```python
from build123d import *

# Parameters (mm, degrees)
SKETCH1_R           = 1.5
SKETCH1_R_2         = 53.34
BOSS_EXTRUDE1_DEPTH = 1.5875
CUT_EXTRUDE3_DEPTH  = 140.70900378


with BuildPart() as part:
    # Sketch1 → Boss-Extrude1 (new body)
    with BuildSketch(Plane(origin=(0, 0, 0), x_dir=(1, 0, 0), z_dir=(0, 1, 0))):
        Polygon((0.047005036, -98.782806148), (-98.782806148, -0.047005036), (-0.047005036, 98.782806148), (98.782806148, 0.047005036), align=None)
        with Locations(Location((-61.346730494, 5.55625, 0), (0, 0, 270))):
            Circle(SKETCH1_R, mode=Mode.SUBTRACT)
        with Locations(Location((-61.346730494, -5.55625, 0), (0, 0, 270))):
            Circle(SKETCH1_R, mode=Mode.SUBTRACT)
        with Locations(Location((-5.55625, -61.346730494, 0), (0, 0, 270))):
            Circle(SKETCH1_R, mode=Mode.SUBTRACT)
        with Locations(Location((5.55625, -61.346730494, 0), (0, 0, 270))):
            Circle(SKETCH1_R, mode=Mode.SUBTRACT)
        with Locations(Location((61.346730494, -5.55625, 0), (0, 0, 270))):
            Circle(SKETCH1_R, mode=Mode.SUBTRACT)
        with Locations(Location((61.346730494, 5.55625, 0), (0, 0, 270))):
            Circle(SKETCH1_R, mode=Mode.SUBTRACT)
        with Locations(Location((5.55625, 61.346730494, 0), (0, 0, 270))):
            Circle(SKETCH1_R, mode=Mode.SUBTRACT)
        with Locations(Location((-5.55625, 61.346730494, 0), (0, 0, 270))):
            Circle(SKETCH1_R, mode=Mode.SUBTRACT)
        with Locations(Location((0, 0, 0), (0, 0, 270))):
            Circle(SKETCH1_R_2, mode=Mode.SUBTRACT)
    extrude(amount=BOSS_EXTRUDE1_DEPTH)

    # Sketch2 → Cut-Extrude3 (cut, through all)
    with BuildSketch(Plane(origin=(0, 1.5875, 0), x_dir=(1, 0, 0), z_dir=(0, 1, 0))):
        Polygon((3.175, 53.34), (3.175, 59.69), (-3.175, 59.69), (-3.175, 53.34), (-3.175, 52.244537665), (3.175, 52.244537665), align=None)
        Polygon((53.34, -3.175), (59.69, -3.175), (59.69, 3.175), (53.34, 3.175), (52.244537665, 3.175), (52.244537665, -3.175), align=None)
        Polygon((-3.175, -53.34), (-3.175, -59.69), (3.175, -59.69), (3.175, -53.34), (3.175, -52.244537665), (-3.175, -52.244537665), align=None)
        Polygon((-53.34, 3.175), (-59.69, 3.175), (-59.69, -3.175), (-53.34, -3.175), (-52.244537665, -3.175), (-52.244537665, 3.175), align=None)
    extrude(amount=-CUT_EXTRUDE3_DEPTH, mode=Mode.SUBTRACT)


solid = part.part
```
Can you work these out from the model? Positions are in its coordinate system, mm. A direction names the side the tool comes from. Coordinates: 2 decimals unless noted, no trailing zeros. Write each loop counter-clockwise with the first axis right and the second up, starting at its lowest first coordinate (ties: lowest second). Pieces come first, ordered by that corner, then holes. Notation, with made-up numbers: M 79.25,12 L 96.25,12 A25 cw 96.25,41 Z; hole C 76,59 d8. An arc over 180 degrees is marked long. Write item = value, one per line. Start each with the question number.
Q1. I'm going to push flat-ended pins straight in: pin 1 (0.5 mm diameter, centred on y = 1, z = 1, fed in from -X); pin 2 (0.8 mm diameter, centred on x = -1, y = 1, fed in from -Z); pin 3 (0.5 mm diameter, centred on x = 56.5, y = 1, fed in from -Z). Where does each tip first touch, or does it pass through?
Q2. If we section it at C-C, the plane y = 1: State how many separate pieces and enclosed holes the cut face has, then the cut area to 3 significant figures.
Q3. If we section it at B-B, the plane z = -33: Write out the boundary of the cut face in (x, y).
Q4. If we section it at A-A, the plane x = -26.5: Write out the boundary of the cut face in (y, z), then the cut area to 3 significant figures.
Q5. If we section it at D-D, the plane z = 83: Write out the boundary of the cut face in (x, y).
Q6. If I drill on L1, parallel to X at y = 1.3, z = 60; L2, parallel to X at y = 1.05, z = -9.5; L3, parallel to Z at x = 55, y = 0.1 (3 decimals), over which ranges is the centre line in solid material (lowest first)? Write a range as [from, to].
Q7. On a 3-axis mill with a long thin cutter (end or side, diameter ignored), from which of +Z, -Z, +X, -X, +Y, -Y can I reach the whole of each face in a straight line? I mean faces 4 (the face through (50.106, 0.783, 48.676)), 5 (the face through (-37.33, 0.78, -38.1)). Say none if no direction works.
Q8. Thinking about a two-plate mould opening in Z: for faces 1 (the face through (48.676, 0.783, -50.106)), 2 (the face through (-38.1, 0.78, 37.33)), 3 (the face through (52, 0, -15)), which applies, released by +Z, released by -Z, zero draft, split by the parting line, or undercut?
Check sheet entries:
q1.pin_1 = -98.08
q1.pin_2 = -98.23
q1.pin_3 = -42.54
q2.separate_pieces = 1
q2.enclosed_holes = 9
q2.area = 10,400 mm²
q3.outline = M -65.77,0 L -41.91,0 L -41.91,1.59 L -65.77,1.59 Z; M 41.91,0 L 65.8,0 L 65.8,1.59 L 41.91,1.59 Z
q4.outline = M 0,-72.3 L 1.59,-72.3 L 1.59,-46.29 L 0,-46.29 Z; M 0,46.29 L 1.59,46.29 L 1.59,72.26 L 0,72.26 Z
q4.area = 82.5 mm²
q5.outline = M -15.75,0 L 15.81,0 L 15.81,1.59 L -15.75,1.59 Z
q6.L1 = [-38.77, -6.22], [-4.9, 4.9], [6.22, 38.79]
q6.L2 = [-89.24, -52.49], [52.49, 89.32]
q6.L3 = [-43.788, -3.175], [3.175, 43.777]
q7.face_4 = +Z, +X, +Y, -Y
q7.face_5 = +Y, -Y
q8.face_1 = released by -Z
q8.face_2 = undercut
q8.face_3 = zero draft
